Source: CAD feature listing. Evaluate the final solid. Frame: model axes, mm. Face numbers are marked on the shaded views. Round coordinates to 2 decimals unless told otherwise and drop trailing zeros. Order: outer loops, then holes, each group sorted by start corner. A loop starts at its lowest first (then second) coordinate and runs counter-clockwise, first axis right, second up.
```python
from build123d import *

# Parameters (mm, degrees)
SKETCH1_W           = 65
SKETCH1_H           = 65
SKETCH1_R           = 2.15
BOSS_EXTRUDE1_DEPTH = 3
SKETCH2_W           = 65
SKETCH2_H           = 65
SKETCH2_R           = 2.15
SKETCH2_W_2         = 50
SKETCH2_H_2         = 50
BOSS_EXTRUDE2_DEPTH = 2
SKETCH3_R           = 1
CUT_EXTRUDE1_DEPTH  = 47.059743812
CHAMFER1_SIZE       = 1.5
SKETCH4_W           = 50
SKETCH4_H           = 50
CUT_EXTRUDE2_DEPTH  = 1


with BuildPart() as part:
    # Sketch1 → Boss-Extrude1 (new body)
    with BuildSketch(Plane.XY):
        Rectangle(SKETCH1_W, SKETCH1_H)
        with Locations((-28.313708499, 28.313708499)):
            Circle(SKETCH1_R, mode=Mode.SUBTRACT)
        with Locations((-28.313708499, -28.313708499)):
            Circle(SKETCH1_R, mode=Mode.SUBTRACT)
        with Locations((28.313708499, -28.313708499)):
            Circle(SKETCH1_R, mode=Mode.SUBTRACT)
        with Locations((28.313708499, 28.313708499)):
            Circle(SKETCH1_R, mode=Mode.SUBTRACT)
    extrude(amount=BOSS_EXTRUDE1_DEPTH)

    # Sketch2 → Boss-Extrude2 (add)
    with BuildSketch(Plane.XY.offset(3)):
        Rectangle(SKETCH2_W, SKETCH2_H)
        with Locations((-28.313708499, -28.313708499)):
            Circle(SKETCH2_R, mode=Mode.SUBTRACT)
        with Locations((28.313708499, -28.313708499)):
            Circle(SKETCH2_R, mode=Mode.SUBTRACT)
        with Locations((-28.313708499, 28.313708499)):
            Circle(SKETCH2_R, mode=Mode.SUBTRACT)
        with Locations((28.313708499, 28.313708499)):
            Circle(SKETCH2_R, mode=Mode.SUBTRACT)
        Rectangle(SKETCH2_W_2, SKETCH2_H_2, mode=Mode.SUBTRACT)
    extrude(amount=BOSS_EXTRUDE2_DEPTH)

    # Sketch3 → Cut-Extrude1 (cut, through all)
    with BuildSketch(Plane.XY.offset(3)):
        with Locations((-20, -20)):
            Circle(SKETCH3_R)
        with Locations((-10, -20)):
            Circle(SKETCH3_R)
        with Locations((0, -20)):
            Circle(SKETCH3_R)
        with Locations((10, -20)):
            Circle(SKETCH3_R)
        with Locations((20, -20)):
            Circle(SKETCH3_R)
        with Locations((-10, -10)):
            Circle(SKETCH3_R)
        with Locations((0, -10)):
            Circle(SKETCH3_R)
        with Locations((10, -10)):
            Circle(SKETCH3_R)
        with Locations((20, -10)):
            Circle(SKETCH3_R)
        with Locations((-10, 0)):
            Circle(SKETCH3_R)
        Circle(SKETCH3_R)
        with Locations((10, 0)):
            Circle(SKETCH3_R)
        with Locations((20, 0)):
            Circle(SKETCH3_R)
        with Locations((-10, 10)):
            Circle(SKETCH3_R)
        with Locations((0, 10)):
            Circle(SKETCH3_R)
        with Locations((10, 10)):
            Circle(SKETCH3_R)
        with Locations((20, 10)):
            Circle(SKETCH3_R)
        with Locations((-10, 20)):
            Circle(SKETCH3_R)
        with Locations((0, 20)):
            Circle(SKETCH3_R)
        with Locations((10, 20)):
            Circle(SKETCH3_R)
        with Locations((20, 20)):
            Circle(SKETCH3_R)
        with Locations((-20, -10)):
            Circle(SKETCH3_R)
        with Locations((-20, 0)):
            Circle(SKETCH3_R)
        with Locations((-20, 10)):
            Circle(SKETCH3_R)
        with Locations((-20, 20)):
            Circle(SKETCH3_R)
    extrude(amount=-CUT_EXTRUDE1_DEPTH, mode=Mode.SUBTRACT)

    # Chamfer1
    chamfer1_edges = [part.edges().sort_by_distance(p)[0] for p in [
        (-30.463708499, 28.313708499, 0),
        (-30.463708499, -28.313708499, 0),
        (26.163708499, -28.313708499, 0),
        (26.163708499, 28.313708499, 0),
    ]]
    chamfer(chamfer1_edges, length=CHAMFER1_SIZE)

    # Sketch4 → Cut-Extrude2 (cut)
    with BuildSketch(Plane(origin=(0, 0, 0), x_dir=(-1, 0, 0), z_dir=(0, 0, -1))):
        Rectangle(SKETCH4_W, SKETCH4_H)
    extrude(amount=-CUT_EXTRUDE2_DEPTH, mode=Mode.SUBTRACT)


solid = part.part
```
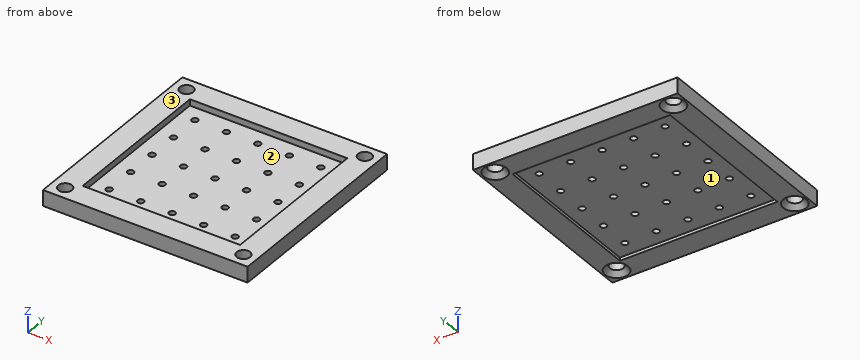
1. Section C-C on y = -18. Return loops of the section in (x, z), plus the area to 3 significant figures.
2. Section A-A on y = 20. State how many separate pieces and enclosed holes the cut face has, plus the area to 3 significant figures.
3. First-contact query: pin 1 (2.5 mm diameter, centred on x = 10, y = -20, fed in from +Z); pin 2 (2.5 mm diameter, centred on x = 20, y = -20, fed in from -Z); pin 3 (1.8 mm diameter, centred on x = -20, y = 10, fed in from +Z). Flat tips, straight axial feed; report the tip coordinate or a pass-through.
4. Pull-direction query (X, two-part tool) for the marked faces 1, 2 and 3; classes: released by +X, released by -X, zero draft, split by the parting line, or undercut.
5. Line query: line 1 along Y through (x, z) = (0, 1.75); line 2 along X through (y, z) = (-19, 3.15). Output: solid intervals per line, ascending.
6. Section D-D on z = 4.25. Return loops of the section in (x, y).
Result:
1. outline: (-32.5, 0) - (-25, 0) - (-25, 1) - (25, 1) - (25, 0) - (32.5, 0) - (32.5, 5) - (25, 5) - (25, 3) - (-25, 3) - (-25, 5) - (-32.5, 5) - close
1. area: 175 mm2
2. separate pieces: 6
2. enclosed holes: 0
2. area: 155 mm2
3. pin 1: stops at z = 3
3. pin 2: stops at z = 1
3. pin 3: passes through
4. face 1: undercut
4. face 2: undercut
4. face 3: zero draft
5. line 1: y = -32.5 to -21, -19 to -11, -9 to -1, 1 to 9, 11 to 19, 21 to 32.5
5. line 2: x = -32.5 to -25, 25 to 32.5
6. outline: (-32.5, -32.5) - (32.5, -32.5) - (32.5, 32.5) - (-32.5, 32.5) - close; hole circle Ø4.3 at (-28.31, -28.31); hole circle Ø4.3 at (-28.31, 28.31); hole (-25, -25) - (25, -25) - (25, 25) - (-25, 25) - close; hole circle Ø4.3 at (28.31, -28.31); hole circle Ø4.3 at (28.31, 28.31)
